Can you work these out from the model? Positions are in its coordinate system, mm. A direction names the side the tool comes from. Coordinates: 2 decimals unless noted, no trailing zeros. Write each loop counter-clockwise with the first axis right and the second up, starting at its lowest first coordinate (ties: lowest second). Pieces come first, ordered by that corner, then holes. Notation, with made-up numbers: (-2.75, 62) -> (2.25, 62) arc R33 ccw to (2.25, 97) -> close; hole circle Ø10 at (24, 54.5). An arc over 180 degrees is marked (long way). Use one line per item in the form item = value.
```python
from build123d import *

# Parameters (mm, degrees)
BOSS_EXTRUDE1_DEPTH = 80
SKETCH4_W           = 20
SKETCH4_H           = 50
BOSS_EXTRUDE2_DEPTH = 50
SKETCH5_R           = 7.5
CUT_EXTRUDE2_DEPTH  = 15
CUT_EXTRUDE3_DEPTH  = 40
CUT_EXTRUDE4_DEPTH  = 40
SKETCH13_R          = 12.5
CUT_EXTRUDE5_DEPTH  = 40
CUT_EXTRUDE6_DEPTH  = 20
FILLET1_R           = 2


with BuildPart() as part:
    # Sketch1 → Boss-Extrude1 (new body)
    with BuildSketch(Plane(origin=(0, 0, 0), x_dir=(0, 0, -1), z_dir=(1, 0, 0))):
        Polygon((-65, -15), (-15, -15), (-23.660254038, -30), (0, -30), (0, 0), (-80, 0), (-80, -30), (-56.339745962, -30), align=None)
    boss_extrude1 = extrude(amount=BOSS_EXTRUDE1_DEPTH)

    # Sketch4 → Boss-Extrude2 (add)
    with BuildSketch(Plane(origin=(0, 0, 0), x_dir=(1, 0, 0), z_dir=(0, 1, 0))):
        with Locations((30, -40)):
            Rectangle(SKETCH4_W, SKETCH4_H)
    boss_extrude2 = extrude(amount=BOSS_EXTRUDE2_DEPTH)

    # Sketch5 → Cut-Extrude2 (cut)
    with BuildSketch(Plane(origin=(0, 0, 0), x_dir=(1, 0, 0), z_dir=(0, 1, 0))):
        with Locations((60, -40)):
            Circle(SKETCH5_R)
    cut_extrude2 = extrude(amount=-CUT_EXTRUDE2_DEPTH, mode=Mode.SUBTRACT)

    # Sketch9 → Cut-Extrude3 (cut)
    with BuildSketch(Plane(origin=(0, 0, 0), x_dir=(0, 0, -1), z_dir=(1, 0, 0))):
        with BuildLine():
            Line((-65, 25), (-65, 50))
            Line((-65, 50), (-40, 50))
            ThreePointArc((-40, 50), (-57.67766953, 42.67766953), (-65, 25))
        make_face()
    cut_extrude3 = extrude(amount=CUT_EXTRUDE3_DEPTH, mode=Mode.SUBTRACT)

    # Sketch11 → Cut-Extrude4 (cut)
    with BuildSketch(Plane(origin=(0, 0, 0), x_dir=(0, 0, -1), z_dir=(1, 0, 0))):
        with BuildLine():
            Line((-15, 25), (-15, 50))
            Line((-15, 50), (-40, 50))
            ThreePointArc((-40, 50), (-22.32233047, 42.67766953), (-15, 25))
        make_face()
    extrude(amount=CUT_EXTRUDE4_DEPTH, mode=Mode.SUBTRACT)

    # Sketch13 → Cut-Extrude5 (cut)
    with BuildSketch(Plane(origin=(0, 0, 0), x_dir=(0, 0, -1), z_dir=(1, 0, 0))):
        with Locations((-40, 25)):
            Circle(SKETCH13_R)
    cut_extrude5 = extrude(amount=CUT_EXTRUDE5_DEPTH, mode=Mode.SUBTRACT)

    # Mirror3: Boss-Extrude1, Boss-Extrude2, Cut-Extrude2, Cut-Extrude3, Cut-Extrude5 across plane
    add(boss_extrude1.mirror(Plane(origin=(0, 0, 0), x_dir=(0, 0, 1), z_dir=(1, 0, 0))))
    add(boss_extrude2.mirror(Plane(origin=(0, 0, 0), x_dir=(0, 0, 1), z_dir=(1, 0, 0))))
    add(cut_extrude2.mirror(Plane(origin=(0, 0, 0), x_dir=(0, 0, 1), z_dir=(1, 0, 0))), mode=Mode.SUBTRACT)
    add(cut_extrude3.mirror(Plane(origin=(0, 0, 0), x_dir=(0, 0, 1), z_dir=(1, 0, 0))), mode=Mode.SUBTRACT)
    add(cut_extrude5.mirror(Plane(origin=(0, 0, 0), x_dir=(0, 0, 1), z_dir=(1, 0, 0))), mode=Mode.SUBTRACT)

    # Sketch17 → Cut-Extrude6 (cut)
    with BuildSketch(Plane(origin=(-20, 0, 0), x_dir=(0, 0, -1), z_dir=(1, 0, 0))):
        with BuildLine():
            Line((-40, 50), (-15, 50))
            Line((-15, 50), (-15, 25))
            ThreePointArc((-15, 25), (-22.32233047, 42.67766953), (-40, 50))
        make_face()
    extrude(amount=-CUT_EXTRUDE6_DEPTH, mode=Mode.SUBTRACT)

    # Fillet1
    fillet1_edges = [part.edges().sort_by_distance(p)[0] for p in [
        (-30, 0, 65),
        (-30, 0, 15),
        (30, 0, 65),
        (30, 0, 15),
    ]]
    fillet(fillet1_edges, radius=FILLET1_R)


solid = part.part
```
Q1. Suppose I cut it at D-D (x = 15). Write out the boundary of the cut face in (y, z).
Return value:
outline = (-30, 0) -> (0, 0) -> (0, 80) -> (-30, 80) -> (-30, 56.34) -> (-15, 65) -> (-15, 15) -> (-30, 23.66) -> close
Q2. Will these pins go through, and if not, where does the flat tip stop? pin 1 (24 mm diameter, centred on x = 60, z = 40, fed in from -Y); pin 2 (15 mm diameter, centred on y = 25, z = 40, fed in from -X); pin 3 (12 mm diameter, centred on x = -16.5, z = 22.5, fed in from +Y); pin 4 (16 mm diameter, centred on x = -28, y = 14.5, fed in from -Z).
Return value:
pin_1 = -15
pin_2 = through
pin_3 = 46.58
pin_4 = 15
Q3. If I drill on line 1 (X direction, y = -7.75, z = 40); line 2 (Y direction, x = 33.5, z = 40); line 3 (X direction, y = 7.5, z = 24), over which ranges is the centre line in solid material (lowest first)? Write a range as from..to.
Return value:
line_1 = -80..-67.5, -52.5..52.5, 67.5..80
line_2 = -15..12.5, 37.5..50
line_3 = -40..-20, 20..40
Q4. Thinking about a two-plate mould opening in Z: for faces 1 (the flat face through (30, 13, 65)), 2 (the flat face through (1.12, -22.395, 19.27)), 3 (the flat face through (1, -15, 40)), 4 (the flat face through (40, 13.5, 34.4)), which applies, released by +Z, released by -Z, zero draft, split by the parting line, or undercut?
Return value:
face_1 = released by +Z
face_2 = undercut
face_3 = undercut
face_4 = zero draft
Q5. Suppose I cut it at B-B (z = 30). Write out the boundary of the cut face in (x, y), then the cut area to 3 significant figures.
Return value:
outline = (-80, -15) -> (80, -15) -> (80, 0) -> (40, 0) -> (40, 17.5) -> (20, 17.5) -> (20, 0) -> (-20, 0) -> (-20, 17.5) -> (-40, 17.5) -> (-40, 0) -> (-80, 0) -> close; (-40, 32.5) -> (-20, 32.5) -> (-20, 47.91) -> (-40, 47.91) -> close; (20, 32.5) -> (40, 32.5) -> (40, 47.91) -> (20, 47.91) -> close
area = 3,720 mm2
Q6. For faces 5 (the flat face through (20, 13.5, 34.4)), 6 (the flat face through (1.12, -22.6, 60.61)), 7 (the flat face through (-30, 13, 15)), 8 (the flat face through (-40, 13.5, 34.4)), which set-ups out of +Z, -Z, +X, -X, +Y, -Y let a thin tool reach every point of the face, with its end or its side?
Return value:
face_5 = +Z, -Z, +Y
face_6 = +X, -X
face_7 = -Z, +X, -X, +Y
face_8 = +Z, -Z, -X, +Y
Q7. Suppose I cut it at A-A (x = 60). Write out the boundary of the cut face in (y, z).
Return value:
outline = (-30, 0) -> (0, 0) -> (0, 32.5) -> (-15, 32.5) -> (-15, 15) -> (-30, 23.66) -> close; (-30, 56.34) -> (-15, 65) -> (-15, 47.5) -> (0, 47.5) -> (0, 80) -> (-30, 80) -> close
Q8. Suppose I cut it at C-C (y = 19). Write out the boundary of the cut face in (x, z).
Return value:
outline = (-40, 15) -> (-20, 15) -> (-20, 29.03) -> (-40, 29.03) -> close; (-40, 50.97) -> (-20, 50.97) -> (-20, 65) -> (-40, 65) -> close; (20, 15) -> (40, 15) -> (40, 29.03) -> (20, 29.03) -> close; (20, 50.97) -> (40, 50.97) -> (40, 65) -> (20, 65) -> close
